Build history of the part. All positions in model axes, mm. A direction names the side the tool comes from. Coordinates: 2 decimals unless noted, no trailing zeros. Loops run counter-clockwise (first coordinate to the right, second up) from the corner with the lowest first, then second, coordinate; pieces in that order, holes last. Notation, with made-up numbers: M -10.75,7.5 L 33.25,7.5 A20 ccw 33.25,45.5 Z; hole C -18.75,-4.5 d8. An arc over 180 degrees is marked long. Write each question's results on one line, items separated by ' | '. Start each with the question number.
from build123d import *

# Parameters (mm, degrees)
SKETCH1_R           = 90.5
SKETCH1_R_2         = 84.5
BOSS_EXTRUDE1_DEPTH = 76.35
CHAMFER1_SIZE       = 6.5
WRAP12_SECTION_W    = 19
WRAP12_SECTION_H    = 69.85
WRAP12_ANGLE        = 32.161608832
CUT_EXTRUDE1_DEPTH  = 63.5
CHAMFER2_SIZE       = 19
CHAMFER5_SIZE       = 15
CHAMFER5_SIZE_2     = 4.019237886
CIRPATTERN6_COUNT   = 4
SKETCH15_R          = 84.5
BOSS_EXTRUDE2_DEPTH = 10


with BuildPart() as part:
    # Sketch1 → Boss-Extrude1 (new body)
    with BuildSketch(Plane.XY):
        Circle(SKETCH1_R)
        Circle(SKETCH1_R_2, mode=Mode.SUBTRACT)
    extrude(amount=BOSS_EXTRUDE1_DEPTH)

    # Chamfer1
    # the kernel refuses this chamfer: 6.5 mm, written as the material it takes off along each edge
    with BuildSketch(Plane(origin=(0, 0, 76.35), x_dir=(1, 0, 0), z_dir=(0, -1, 0))) as chamfer1_piece_1:
        Polygon((90.5, -CHAMFER1_SIZE), (90.5 - CHAMFER1_SIZE, 0), (90.5, 0), align=None)
    revolve(axis=Axis((0, 0, 76.35), (0, 0, 1)), mode=Mode.SUBTRACT)

    # Wrap12 section (on wrap section) → Wrap12 (revolve)
    with BuildSketch(Plane(origin=(0, 0, 0), x_dir=(0.9608717281441653, 0.276993722046629, 0), z_dir=(-0.276993722046629, 0.9608717281441653, 0))):
        with Locations((100, -34.925)):
            Rectangle(WRAP12_SECTION_W, WRAP12_SECTION_H)
    revolve(axis=Axis((0, 0, 0), (0, 0, -1)), revolution_arc=WRAP12_ANGLE)

    # Sketch12 → Cut-Extrude1 (cut)
    with BuildSketch(Plane.XY.offset(69.85)):
        Polygon((122.706651928, -0.201195148), (122.706651928, 3.507927311), (97.67138598, 3.507927311), (97.67138598, 10.503148948), (90.66864355, 10.503148948), (90.66864355, -10.492123054), (97.67138598, -10.492123054), (97.67138598, -3.492123054), (122.706651928, -3.70406248), align=None)
    extrude(amount=-CUT_EXTRUDE1_DEPTH, mode=Mode.SUBTRACT)

    # Chamfer2
    # the kernel refuses this chamfer: 19 mm, written as the material it takes off along each edge
    with BuildSketch(Plane(origin=(105.215515497, -30.330600038, 118.711976771), x_dir=(-0.9608722876451651, 0.27699178116967144, 0), z_dir=(0, 0, -1))) as chamfer2_piece_1_section:
        with BuildLine():
            Line((CHAMFER2_SIZE, 0), (1.420369251, 17.579630749))
            ThreePointArc((1.420369251, 17.579630749), (0.375784571, 9.063973019), (0, 0))
            Line((0, 0), (CHAMFER2_SIZE, 0))
        make_face()
    chamfer2_piece_1 = extrude(amount=167.573953543, mode=Mode.PRIVATE)
    chamfer2_piece_1 = chamfer2_piece_1 - Plane(origin=(0, 0, 118.711976771), x_dir=(1, 0, 0), z_dir=(0, 0, -1)) * Cylinder(90.5, 412, mode=Mode.PRIVATE)
    add(chamfer2_piece_1, mode=Mode.SUBTRACT)
    with BuildSketch(Plane(origin=(105.215454232, 30.330812564, 118.711976771), x_dir=(-0.9608717281441654, -0.2769937220466291, 0), z_dir=(0, 0, -1))) as chamfer2_piece_2_section:
        with BuildLine():
            Line((CHAMFER2_SIZE, 0), (1.420369251, -17.579630749))
            ThreePointArc((1.420369251, -17.579630749), (0.375784571, -9.063973019), (0, 0))
            Line((0, 0), (CHAMFER2_SIZE, 0))
        make_face()
    chamfer2_piece_2 = extrude(amount=167.573953543, mode=Mode.PRIVATE)
    chamfer2_piece_2 = chamfer2_piece_2 - Plane(origin=(0, 0, 118.711976771), x_dir=(1, 0, 0), z_dir=(0, 0, -1)) * Cylinder(90.5, 412, mode=Mode.PRIVATE)
    add(chamfer2_piece_2, mode=Mode.SUBTRACT)

    # Chamfer5
    # the kernel refuses this chamfer: 15, 4.019237886 mm, written as the material it takes off along each edge
    with BuildSketch(Plane(origin=(52.865116584, 43.903567605, 69.85), x_dir=(0, 0, -1), z_dir=(0.8753030540266438, -0.483574775615551, 0))) as chamfer5_piece_1_section:
        Polygon((CHAMFER5_SIZE, 0), (0, -CHAMFER5_SIZE_2), (0, 0), align=None)
    chamfer5_piece_1 = extrude(amount=102.762999332, mode=Mode.PRIVATE)
    chamfer5_piece_1 = chamfer5_piece_1 - Plane(origin=(0, 0, 69.85), x_dir=(1, 0, 0), z_dir=(0, 0, -1)) * Cylinder(90.5, 266, mode=Mode.PRIVATE)
    add(chamfer5_piece_1, mode=Mode.SUBTRACT)
    with BuildSketch(Plane(origin=(52.865205265, -43.903460822, 69.85), x_dir=(0, 0, -1), z_dir=(0.8753020772463168, 0.48357654364979585, 0))) as chamfer5_piece_2_section:
        Polygon((CHAMFER5_SIZE, 0), (0, CHAMFER5_SIZE_2), (0, 0), align=None)
    chamfer5_piece_2 = extrude(amount=102.762999332, mode=Mode.PRIVATE)
    chamfer5_piece_2 = chamfer5_piece_2 - Plane(origin=(0, 0, 69.85), x_dir=(1, 0, 0), z_dir=(0, 0, -1)) * Cylinder(90.5, 266, mode=Mode.PRIVATE)
    add(chamfer5_piece_2, mode=Mode.SUBTRACT)


with BuildPart() as cirpattern6_1:
    # CirPattern6: pattern copy
    add(part.part.rotate(Axis((0, 0, 0), (0, 0, 1)), 1 * 360 / CIRPATTERN6_COUNT))


with BuildPart() as cirpattern6_2:
    # CirPattern6: pattern copy
    add(part.part.rotate(Axis((0, 0, 0), (0, 0, 1)), 2 * 360 / CIRPATTERN6_COUNT))


with BuildPart() as cirpattern6_3:
    # CirPattern6: pattern copy
    add(part.part.rotate(Axis((0, 0, 0), (0, 0, 1)), 3 * 360 / CIRPATTERN6_COUNT))


with BuildPart() as part_1:
    add(part.part)

    add(cirpattern6_1.part)  # Boss-Extrude2 merges CirPattern6_1

    add(cirpattern6_2.part)  # Boss-Extrude2 merges CirPattern6_2

    add(cirpattern6_3.part)  # Boss-Extrude2 merges CirPattern6_3
    # Sketch15 → Boss-Extrude2 (add)
    with BuildSketch(Plane(origin=(0, 0, 0), x_dir=(-1, 0, 0), z_dir=(0, 0, -1))):
        Circle(SKETCH15_R)
    extrude(amount=-BOSS_EXTRUDE2_DEPTH)


solid = part_1.part
1. Wall check: line 1 along X through (y, z) = (-0.5, 47); line 2 along Z through (x, y) = (-65.5, 29.5). Give the ranges that are in metal, low to high.
2. Band-saw the part on C-C, the plane x = 93.5. List the corners of the cut face in (y, z), plus the area to 3 significant figures.
3. Band-saw the part on A-A, the plane x = 0. List the corners of the cut face in (y, z), plus the area to 3 significant figures.
4. Pin check, flat tips, straight feed: pin 1 (7.5 mm diameter, centred on x = 7, z = 51, fed in from -Y); pin 2 (20.5 mm diameter, centred on x = 99.5, y = -3.5, fed in from +Z); pin 3 (3 mm diameter, centred on x = 55.5, z = 10.5, fed in from -Y). Stop position of each tip, or through.
5. Which spindle directions (+Z, -Z, +X, -X, +Y, -Y) get a long thin tool onto all of the face, cutting with end or side? Do faces 4 (the flat face through (1, 1, 10)), 5 (the flat face through (97.69, -19.14, 27.81)). Say none if no direction does.
6. Mould opens along Y. For faces 1 (the flat face through (2, 2, 0)), 2 (the flat face through (7, 97.671, 39)), 3 (the flat face through (97.69, 19.14, 27.81)) say: +Y half, -Y half, draft (parallel to the pull), parting line (faces both ways), or undercut.
Checked values:
1) line 1: -90.67 to -84.5, 84.5 to 90.67 | line 2: 0 to 10
2) outline: M -21.45,0 L 21.45,0 L 21.45,54.85 L 16.86,69.85 L 10.5,69.85 L 10.5,6.35 L -10.49,6.35 L -10.49,69.85 L -16.86,69.85 L -21.45,54.85 Z | area: 1,600 mm²
3) outline: M -109.5,0 L 109.5,0 L 109.5,6.35 L 90.67,6.35 L 90.67,69.85 L 90.5,69.85 L 84.5,75.85 L 84.5,10 L -84.5,10 L -84.5,75.85 L -90.5,69.85 L -90.67,69.85 L -90.67,6.35 L -109.5,6.35 Z | area: 2,830 mm²
4) pin 1: y = -109.44 | pin 2: z = 71.04 | pin 3: y = -72.62
5) face 4: +Z | face 5: +Z, -Z, +X, -Y
6) face 1: draft | face 2: undercut | face 3: +Y half
